Design review of the part built by this model. Coordinates are the model's own, in mm. Give positions to 0.01 mm unless a question says otherwise; leave off trailing zeros. Order: outer loops, then holes, each group sorted by start corner. A loop starts at its lowest first (then second) coordinate and runs counter-clockwise, first axis right, second up. Notation, with made-up numbers: (-1.75, -15.5) -> (32.25, -15.5) arc R5 ccw to (32.25, -11.5) -> close; hole circle Ø1 at (-9, -4.75). An arc over 180 degrees is marked (long way). One line per item, written item: value. Start each with the question number.
1) Consider section A-A (z = -3.5). State the section outline as (x, y) points (3 decimals).
2) The part is to be moulded in two halves that separate along Z. For faces 1 (the face through (8, 3.175, -1)), 2 (the face through (25.973, 1.565, -27.874)), 3 (the face through (3.855, 1.565, 31.755)), say which applies: released by +Z, released by -Z, zero draft, split by the parting line, or undercut.
3) Wall thickness on line 1 along X through (y, z) = (1.9, -2); line 2 along X through (y, z) = (0.85, -1); line 3 along Z through (x, y) = (-30, 1.85): over which ranges is each line inside the solid? List them lowest first. Write a range as from..to.
4) Consider section B-B (z = 8). State the section outline as (x, y) points (3 decimals), plus the area to 3 significant figures.
5) For pin 1 (1 mm diameter, centred on x = -6.5, y = 0.5, fed in from -Z); pin 2 (1.5 mm diameter, centred on x = -19, y = 1, fed in from +Z); pin 3 (1.5 mm diameter, centred on x = 4.5, y = 1, fed in from +Z), all flat-tipped, find the tip position at first contact; note any pin that passes through.
6) Consider section C-C (z = -13). State the section outline as (x, y) points (3 decimals), plus the area to 3 significant figures.
from build123d import *

# Parameters (mm, degrees)
SKETCH1_R           = 6.604
BOSS_EXTRUDE1_DEPTH = 3.175


with BuildPart() as part:
    # Sketch1 → Boss-Extrude1 (new body)
    with BuildSketch(Plane(origin=(0, 0, 0), x_dir=(1, 0, 0), z_dir=(0, 1, 0))):
        with BuildLine():
            ThreePointArc((0, -36.208877371), (3.945014404, -31.74323173), (8.863107106, -35.107380035))
            ThreePointArc((8.863107106, -35.107380035), (11.19297859, -36.418775793), (12.384165428, -34.025214873))
            ThreePointArc((12.384165428, -34.025214873), (14.563925591, -28.479606225), (20.336027496, -29.958784791))
            ThreePointArc((20.336027496, -29.958784791), (22.973914302, -30.39423073), (23.274617735, -27.737609302))
            ThreePointArc((23.274617735, -27.737609302), (23.42621241, -21.780919895), (29.356122842, -21.196717957))
            ThreePointArc((29.356122842, -21.196717957), (31.98385689, -20.703692869), (31.357807646, -18.104438686))
            ThreePointArc((31.357807646, -18.104438686), (29.462952279, -12.455133173), (34.835436523, -9.878014107))
            ThreePointArc((34.835436523, -9.878014107), (37.136074307, -8.515984094), (35.658783163, -6.287605571))
            ThreePointArc((35.658783163, -6.287605571), (31.946025276, -1.627073572), (36.113082444, 2.632124028))
            ThreePointArc((36.113082444, 2.632124028), (37.809133091, 4.698878045), (35.658783163, 6.287605571))
            ThreePointArc((35.658783163, 6.287605571), (30.575936152, 9.397235114), (33.034957649, 14.824789159))
            ThreePointArc((33.034957649, 14.824789159), (33.921852422, 17.346986144), (31.357807646, 18.104438686))
            ThreePointArc((31.357807646, 18.104438686), (25.517937875, 19.288098557), (25.972329417, 25.229365928))
            ThreePointArc((25.972329417, 25.229365928), (25.943095717, 27.902791699), (23.274617735, 27.737609302))
            ThreePointArc((23.274617735, 27.737609302), (17.382099685, 26.852532653), (15.777054948, 32.590908819))
            ThreePointArc((15.777054948, 32.590908819), (14.835218789, 35.093108775), (12.384165428, 34.025214873))
            ThreePointArc((12.384165428, 34.025214873), (7.149723742, 31.178155009), (3.678834807, 36.021507116))
            ThreePointArc((3.678834807, 36.021507116), (1.937995531, 38.050679013), (0, 36.208877371))
            ThreePointArc((0, 36.208877371), (-3.945014404, 31.74323173), (-8.863107106, 35.107380035))
            ThreePointArc((-8.863107106, 35.107380035), (-11.19297859, 36.418775793), (-12.384165428, 34.025214873))
            ThreePointArc((-12.384165428, 34.025214873), (-14.563925591, 28.479606225), (-20.336027496, 29.958784791))
            ThreePointArc((-20.336027496, 29.958784791), (-22.973914302, 30.39423073), (-23.274617735, 27.737609302))
            ThreePointArc((-23.274617735, 27.737609302), (-23.42621241, 21.780919895), (-29.356122842, 21.196717957))
            ThreePointArc((-29.356122842, 21.196717957), (-31.98385689, 20.703692869), (-31.357807646, 18.104438686))
            ThreePointArc((-31.357807646, 18.104438686), (-29.462952279, 12.455133173), (-34.835436523, 9.878014107))
            ThreePointArc((-34.835436523, 9.878014107), (-37.136074307, 8.515984094), (-35.658783163, 6.287605571))
            ThreePointArc((-35.658783163, 6.287605571), (-31.946025276, 1.627073572), (-36.113082444, -2.632124028))
            ThreePointArc((-36.113082444, -2.632124028), (-37.809133091, -4.698878045), (-35.658783163, -6.287605571))
            ThreePointArc((-35.658783163, -6.287605571), (-30.575936152, -9.397235114), (-33.034957649, -14.824789159))
            ThreePointArc((-33.034957649, -14.824789159), (-33.921852422, -17.346986144), (-31.357807646, -18.104438686))
            ThreePointArc((-31.357807646, -18.104438686), (-25.517937875, -19.288098557), (-25.972329417, -25.229365928))
            ThreePointArc((-25.972329417, -25.229365928), (-25.943095717, -27.902791699), (-23.274617735, -27.737609302))
            ThreePointArc((-23.274617735, -27.737609302), (-17.382099685, -26.852532653), (-15.777054948, -32.590908819))
            ThreePointArc((-15.777054948, -32.590908819), (-14.835218789, -35.093108775), (-12.384165428, -34.025214873))
            ThreePointArc((-12.384165428, -34.025214873), (-7.149723742, -31.178155009), (-3.678834807, -36.021507116))
            ThreePointArc((-3.678834807, -36.021507116), (-1.937995531, -38.050679013), (0, -36.208877371))
        make_face()
        with Locations(Location((0, 0, 0), (0, 0, 270))):  # turned: the seam where the file's is
            Circle(SKETCH1_R, mode=Mode.SUBTRACT)
    extrude(amount=BOSS_EXTRUDE1_DEPTH)


solid = part.part
Checked values:
1. outline: (-32.251, 0) -> (-5.6, 0) -> (-5.6, 3.175) -> (-32.251, 3.175) -> close; (5.6, 0) -> (37.547, 0) -> (37.547, 3.175) -> (5.6, 3.175) -> close
2. face 1: zero draft
2. face 2: undercut
2. face 3: released by +Z
3. line 1: x = -31.94..-6.29, 6.29..34.12
3. line 2: x = -32.02..-6.53, 6.53..32.96
3. line 3: z = -21.49..-16.9, -11.52..17.59
4. outline: (-31.292, 0) -> (37.18, 0) -> (37.18, 3.175) -> (-31.292, 3.175) -> close
4. area: 217 mm^2
5. pin 1: stops at z = -32.47
5. pin 2: stops at z = 26.42
5. pin 3: stops at z = 31.77
6. outline: (-29.273, 0) -> (30.998, 0) -> (30.998, 3.175) -> (-29.273, 3.175) -> close
6. area: 191 mm^2
